```python
from build123d import *

# Parameters (mm, degrees)
SKETCH_W               = 150
SKETCH_H               = 150
PAD_DEPTH              = 2
POCKET_DEPTH           = 2.001
LINEARPATTERN_COUNT    = 13
LINEARPATTERN_PITCH    = 10.833333
SKETCH002_W            = 154
SKETCH002_H            = 154
SKETCH002_W_2          = 150
SKETCH002_H_2          = 150
PAD001_DEPTH           = 50
POCKET001_DEPTH        = 152
POCKET001_DEPTH_BACK   = 2
POCKET002_DEPTH        = 2
POCKET002_DEPTH_BACK   = 152
LINEARPATTERN001_COUNT = 3
LINEARPATTERN001_PITCH = 62.5
LINEARPATTERN002_COUNT = 3
LINEARPATTERN002_PITCH = 62.5
POCKET003_DEPTH        = 152
POCKET003_DEPTH_BACK   = 2
POCKET004_DEPTH        = 2
POCKET004_DEPTH_BACK   = 152


with BuildPart() as part:
    # Sketch → Pad (new body)
    with BuildSketch(Plane.XY):
        with Locations((75, 75)):
            Rectangle(SKETCH_W, SKETCH_H)
    extrude(amount=PAD_DEPTH)

    # Sketch001 → Pocket (cut, through all)
    with BuildSketch(Plane.XY):
        with BuildLine():
            ThreePointArc((11.6, 140), (10, 141.6), (8.4, 140))
            Line((8.4, 140), (8.4, 10))
            ThreePointArc((8.4, 10), (10, 8.4), (11.6, 10))
            Line((11.6, 140), (11.6, 10))
        make_face()
    pocket = extrude(amount=POCKET_DEPTH, mode=Mode.SUBTRACT)

    # LinearPattern: Pocket ×13
    with Locations(*[(i * LINEARPATTERN_PITCH, 0, 0) for i in range(1, LINEARPATTERN_COUNT)]):
        add(pocket, mode=Mode.SUBTRACT)

    # Sketch002 → Pad001 (join)
    with BuildSketch(Plane.XY):
        with Locations((75, 75)):
            Rectangle(SKETCH002_W, SKETCH002_H)
        with Locations((75, 75)):
            Rectangle(SKETCH002_W_2, SKETCH002_H_2, mode=Mode.SUBTRACT)
    extrude(amount=PAD001_DEPTH)

    # Sketch003 → Pocket001 (cut, two sides)
    with BuildSketch(Plane.XZ) as pocket001_sk:
        with BuildLine():
            ThreePointArc((10, 46.6), (8.4, 45), (10, 43.4))
            Line((10, 43.4), (12, 43.4))
            ThreePointArc((12, 43.4), (13.6, 45), (12, 46.6))
            Line((10, 46.6), (12, 46.6))
        make_face()
    pocket001 = extrude(amount=-POCKET001_DEPTH, mode=Mode.SUBTRACT) + extrude(pocket001_sk.sketch, amount=POCKET001_DEPTH_BACK, mode=Mode.SUBTRACT)

    # Sketch004 → Pocket002 (cut, two sides)
    with BuildSketch(Plane.YZ) as pocket002_sk:
        with BuildLine():
            ThreePointArc((10, 43.4), (11.6, 45), (10, 46.6))
            Line((10, 46.6), (8, 46.6))
            ThreePointArc((8, 46.6), (6.4, 45), (8, 43.4))
            Line((10, 43.4), (8, 43.4))
        make_face()
    pocket002 = extrude(amount=-POCKET002_DEPTH, mode=Mode.SUBTRACT) + extrude(pocket002_sk.sketch, amount=POCKET002_DEPTH_BACK, mode=Mode.SUBTRACT)

    # LinearPattern001: Pocket001 ×3
    with Locations(*[(i * LINEARPATTERN001_PITCH, 0, 0) for i in range(1, LINEARPATTERN001_COUNT)]):
        add(pocket001, mode=Mode.SUBTRACT)

    # LinearPattern002: Pocket002 ×3
    with Locations(*[(0, i * LINEARPATTERN002_PITCH, 0) for i in range(1, LINEARPATTERN002_COUNT)]):
        add(pocket002, mode=Mode.SUBTRACT)

    # Sketch005 → Pocket003 (cut, two sides)
    with BuildSketch(Plane.XZ) as pocket003_sk:
        Polygon((20, 10), (60, 10), (40, 30), align=None)
    extrude(amount=-POCKET003_DEPTH, mode=Mode.SUBTRACT)
    extrude(pocket003_sk.sketch, amount=POCKET003_DEPTH_BACK, mode=Mode.SUBTRACT)

    # Sketch006 → Pocket004 (cut, two sides)
    with BuildSketch(Plane.YZ) as pocket004_sk:
        Polygon((20, 10), (60, 10), (40, 30), align=None)
    extrude(amount=-POCKET004_DEPTH, mode=Mode.SUBTRACT)
    extrude(pocket004_sk.sketch, amount=POCKET004_DEPTH_BACK, mode=Mode.SUBTRACT)


solid = part.part
```
CAD build for the part. Positions are in the model's coordinates, mm. A direction names the side the tool comes from. Round coordinates to 2 decimals unless told otherwise and drop trailing zeros. Write each loop counter-clockwise with the first axis right and the second up, starting at its lowest first coordinate (ties: lowest second). Pieces come first, ordered by that corner, then holes. Notation, with made-up numbers: (-27.5, -32.5) -> (-0.5, -32.5) arc R9 ccw to (-0.5, -23.5) -> close; hole circle Ø1 at (42.5, 21). An arc over 180 degrees is marked (long way). Answer in a Markdown table with one row per item. Add a question column.
Item 1: Mould opens along X. For faces 5 (the face through (-2, 74, 25)), 6 (the face through (74, 0, 26)), 7 (the face through (-1, 30, 20)) say: pulls with the +X half, pulls with the -X half, needs draft (parallel to the pull), parting line crosses it, or undercut.
Item 2: Saw through at C-C, the plane x = 113. Write the cut outline in (y, z), then the cut area to 3 significant figures.
Item 3: Which spindle directions (+Z, -Z, +X, -X, +Y, -Y) get a long thin tool onto all of the face, cutting with end or side? Do faces 1 (the face through (152, 74, 25)), 2 (the face through (-1, 50, 20)), 3 (the face through (30, 151, 20)), 4 (the face through (150, 74, 26)). Say none if no direction does.
Item 4: Saw through at B-B, the plane y = 79. Count the separate pieces of the cut face and the enclosed holes in it, then the cut area to 3 significant figures.
Item 5: Saw through at A-A, the plane z = 28. Write the cut outline in (x, y), then the cut area to 3 significant figures.
Item 6: Drill centre lines: line 1 (X direction, y = 140, z = 4); line 2 (Z direction, x = 91, y = 113). Where is each one in solid material? Low to high. Write a range as from..to.
Findings below:
| question | item | result |
|---|---|---|
| 1 | face 5 | pulls with the -X half |
| 1 | face 6 | undercut |
| 1 | face 7 | needs draft |
| 2 | outline | (-2, 0) -> (152, 0) -> (152, 50) -> (150, 50) -> (150, 2) -> (0, 2) -> (0, 50) -> (-2, 50) -> close |
| 2 | area | 500 mm^2 |
| 3 | face 1 | +Z, -Z, +X, +Y, -Y |
| 3 | face 2 | +X, -X |
| 3 | face 3 | +Y, -Y |
| 3 | face 4 | +Z |
| 4 | separate pieces | 14 |
| 4 | enclosed holes | 0 |
| 4 | area | 417 mm^2 |
| 5 | outline | (-2, -2) -> (38, -2) -> (38, 0) -> (0, 0) -> (0, 38) -> (-2, 38) -> close; (-2, 42) -> (0, 42) -> (0, 150) -> (38, 150) -> (38, 152) -> (-2, 152) -> close; (42, -2) -> (152, -2) -> (152, 38) -> (150, 38) -> (150, 0) -> (42, 0) -> close; (42, 150) -> (150, 150) -> (150, 42) -> (152, 42) -> (152, 152) -> (42, 152) -> close |
| 5 | area | 1,180 mm^2 |
| 6 | line 1 | x = -2..0, 150..152 |
| 6 | line 2 | z = 0..2 |
